Autodesk Inventor part; units mm, degrees
ref_plane "YZ Plane" through (0, 0, 0) normal (1, 0, 0) x (0, 1, 0)
ref_plane "XZ Plane" through (0, 0, 0) normal (0, 1, 0) x (-1, 0, 0)
ref_plane "XY Plane" through (0, 0, 0) normal (0, 0, 1) x (1, 0, 0)
sketch "Sketch1" plane through (0, 0, 0) normal (0, 1, 0) x (-1, 0, 0)
  line L0 (0, 0) -> (-95, 0)
  line L1 (-95, 0) -> (-95, -55)
  line L2 (-95, -55) -> (0, -55)
  line L3 (0, -55) -> (0, 0)
  dimension "d0" = 55
  dimension "d1" = 95
extrude "Extrusion1" add sketch "Sketch1" along normal blind 6.5
sketch "Sketch3" plane through (0, 6.5, 0) normal (0, 1, 0) x (1, 0, 0)
  line L0 (0, 0) -> (95, 0)
  line L1 (95, 55) -> (0, 55)
  line L2 (0, 55) -> (0, 0)
  line L3 (0, 49) -> (-4.5, 49)
  line L4 (-6.5, 47) -> (-6.5, 43)
  line L5 (-4.5, 41) -> (0, 41)
  line L6 (0, 41) -> (0, 49)
  line L7 (47.5, 55) -> (47.5, 0) construction
  line L8 (0, 14) -> (-4.5, 14)
  line L9 (-6.5, 12) -> (-6.5, 8)
  line L10 (-4.5, 6) -> (0, 6)
  line L11 (0, 6) -> (0, 14)
  arc A0 (-4.5, 49) -> (-6.5, 47) centre (-4.5, 47) ccw
  arc A1 (-6.5, 43) -> (-4.5, 41) centre (-4.5, 43) ccw
  arc A2 (-4.5, 14) -> (-6.5, 12) centre (-4.5, 12) ccw
  arc A3 (-6.5, 8) -> (-4.5, 6) centre (-4.5, 8) ccw
  line L12 (95, 49) -> (99.5, 49)
  line L13 (101.5, 47) -> (101.5, 43)
  line L14 (99.5, 41) -> (95, 41)
  line L15 (95, 41) -> (95, 49)
  line L16 (95, 14) -> (99.5, 14)
  line L17 (101.5, 12) -> (101.5, 8)
  line L18 (99.5, 6) -> (95, 6)
  line L19 (95, 6) -> (95, 14)
  arc A4 (101.5, 47) -> (99.5, 49) centre (99.5, 47) ccw
  arc A5 (99.5, 41) -> (101.5, 43) centre (99.5, 43) ccw
  arc A6 (101.5, 12) -> (99.5, 14) centre (99.5, 12) ccw
  arc A7 (99.5, 6) -> (101.5, 8) centre (99.5, 8) ccw
  dimension "d13" = 2
  dimension "d14" = 8
  dimension "d15" = 8
  dimension "d16" = 6.5
  dimension "d17" = 6
  dimension "d18" = 6
extrude "Extrusion3" add sketch "Sketch3" against normal blind 6.5
sketch "Sketch4" plane through (0, 0, 0) normal (0, -1, 0) x (1, 0, 0)
  line L0 (0, -41) -> (0, -14)
  line L1 (16.3, -25.25) -> (16.3, -29.75)
  line L2 (0, -29.75) -> (0, -25.25)
  line L3 (5, -22.75) -> (12.3, -22.75)
  line L4 (12.3, -32.25) -> (5, -32.25)
  line L5 (0, -25.25) -> (5, -25.25)
  line L6 (12.3, -25.25) -> (16.3, -25.25)
  line L7 (16.3, -29.75) -> (12.3, -29.75)
  line L8 (5, -29.75) -> (0, -29.75)
  line L9 (5, -32.25) -> (5, -29.75)
  line L10 (5, -25.25) -> (5, -22.75)
  line L11 (12.3, -22.75) -> (12.3, -25.25)
  line L12 (12.3, -29.75) -> (12.3, -32.25)
  point P0 (0, -27.5)
  dimension "d21" = 4.5
  dimension "d22" = 5
  dimension "d23" = 4
  dimension "d24" = 7.3
  dimension "d25" = 2.5
extrude "Extrusion4" cut sketch "Sketch4" against normal through all
equation "\"d18\" = d17"
properties part number "spool_brace" material "Plywood, Finish"
Geometry: final body of the model. Coordinates: model frame, mm. A direction names the side the tool comes from. Coordinates: 2 decimals unless noted, no trailing zeros. Loops run counter-clockwise (first coordinate to the right, second up) from the corner with the lowest first, then second, coordinate; pieces in that order, holes last. Notation, with made-up numbers: (-35.75, -10) - (-22.75, -10) arc R16 cw to (-22.75, 4) - close; hole circle Ø2 at (25, -20.5). An arc over 180 degrees is marked (long way). One line per question, with ' | ' between items. Start each with the question number.
(1) Reachability of faces 4 (the flat face through (3, 3, -29.75)), 5 (the flat face through (12.3, 3, -24)), 6 (the flat face through (95, 3, -3)), 7 (the flat face through (48, 6.5, -27)) from +Z, -Z, +X, -X, +Y, -Y: full face, straight path, thin tool, end or side. Return the list, or none.
(2) Ray query, L1, parallel to X at y = 5.5, z = -31; L2, parallel to X at y = 3.25, z = -53; L3, parallel to X at y = 0.75, z = -29. Return the intervals inside material, ascending. Write a range as from..to.
(3) Draft query along Z for faces 1 (the flat face through (101.5, 3, -10)), 2 (the flat face through (9, 3, -22.75)), 3 (the flat face through (97, 3, -49)). Return one class per face: +Z half, -Z half, draft (parallel to the pull), parting line (faces both ways), or undercut.
(4) Cut plane B-B on z = -21. Output: boundary loops of the cut face in (x, y).
(5) Cut plane A-A on z = -31. Output: boundary loops of the cut face in (x, y), and give its area (3 significant figures).
(6) First-contact query: pin 1 (1.3 mm diameter, centred on x = 97, y = 3, fed in from +Z); pin 2 (1 mm diameter, centred on x = 71, z = -8.5, fed in from -Y); pin 3 (2 mm diameter, centred on y = 5, z = -21, fed in from -X); pin 4 (1.8 mm diameter, centred on y = 2.5, z = -51.5, fed in from +X). Flat tips, straight axial feed; report the tip coordinate or a pass-through.
Here are the results:
1) face 4: -X, +Y, -Y | face 5: +Y, -Y | face 6: +Z, +X, +Y, -Y | face 7: +Z, -Z, +X, -X, +Y
2) L1: 0..5, 12.3..95 | L2: 0..95 | L3: 16.3..95
3) face 1: draft | face 2: undercut | face 3: -Z half
4) outline: (0, 0) - (95, 0) - (95, 6.5) - (0, 6.5) - close
5) outline: (0, 0) - (5, 0) - (5, 6.5) - (0, 6.5) - close; (12.3, 0) - (95, 0) - (95, 6.5) - (12.3, 6.5) - close | area: 570 mm²
6) pin 1: z = -6 | pin 2: y = 0 | pin 3: x = 0 | pin 4: x = 95
